Part model, mm, in its own coordinate system. A direction names the side the tool comes from. Coordinates: 2 decimals unless noted, no trailing zeros. Use a Markdown table: item, result. Add a question column.
Q1. Mould opens along Z. For faces 3 (the flat face through (250, -30, 381)), 4 (the conical face through (198.9, -36.7, 160.1)), 5 (the flat face through (250, -30, 0)), 6 (the flat face through (508, -30, 188)) say: released by +Z, released by -Z, zero draft, split by the parting line, or undercut.
Q2. Wall check: L1, parallel to X at y = -44, z = 160; L2, parallel to Z at x = 200, y = -54. Give the ranges that are in metal, low to high. Write a range as from..to.
Q3. Tool access for faces 1 (the flat face through (250, 0, 191)), 2 (the cylindrical face through (196.452, -49.86, 165.565)): list every direction of +Z, -Z, +X, -X, +Y, -Y with a clear straight run to the whole face (end or side of a thin tool).
from build123d import *

# Parameters (mm, degrees)
F0_W     = 508
F0_H     = 381
F1_DEPTH = 60
F3_D     = 13.2
F3_DEPTH = 20
F3_TIP   = 3.9656800856
F4_R     = 5


with BuildPart() as f1:
    # F0 (on Front) → F1 (new body)
    with BuildSketch(Plane.XZ):
        with Locations((254, 190.5)):
            Rectangle(F0_W, F0_H)
    extrude(amount=F1_DEPTH)

    # F3
    with Locations(Plane.XZ.offset(60)):
        with Locations((200, 160)):
            Hole(F3_D / 2, depth=F3_DEPTH)
            with Locations((0, 0, -(F3_DEPTH + F3_TIP / 2))):  # 118° drill point
                Cone(0, F3_D / 2, F3_TIP, mode=Mode.SUBTRACT)

    # F4
    f4_edges = [f1.edges().sort_by_distance(p)[0] for p in [
        (254, -60, 381),
        (254, 0, 381),
    ]]
    fillet(f4_edges, radius=F4_R)


solid = f1.part
Recorded:
| question | item | result |
|---|---|---|
| 1 | face 3 | released by +Z |
| 1 | face 4 | undercut |
| 1 | face 5 | released by -Z |
| 1 | face 6 | zero draft |
| 2 | L1 | 0..193.4, 206.6..508 |
| 2 | L2 | 0..153.4, 166.6..381 |
| 3 | face 1 | +Z, -Z, +X, -X, +Y |
| 3 | face 2 | -Y |
